Source: CAD feature listing. Evaluate the final solid. Frame: model axes, mm. A direction names the side the tool comes from. Give positions to 0.01 mm unless a question says otherwise; leave off trailing zeros. Loops run counter-clockwise (first coordinate to the right, second up) from the corner with the lowest first, then second, coordinate; pieces in that order, holes last. Notation, with made-up numbers: (48.5, -33) -> (103.5, -33) arc R28 ccw to (103.5, 2) -> close; hole circle Ø6 at (-36.5, 71). An arc over 180 degrees is marked (long way). Put each result on its own line as item: value.
Autodesk Fusion 360 part; units mm, degrees
sketch "Sketch1" plane through (0, 0, 0) normal (0, 1, 0) x (1, 0, 0)
  circle A0 centre (0, 0) radius 80
  dimension "d1" = 160
extrude "Extrude1" add sketch "Sketch1" along normal blind 10 makes body 1
fillet "Fillet1" radius 4 1 edges at (-74.5862, 10, 28.9292) on bodies 1
sketch "Sketch2" plane through (0, 0, 0) normal (0, 1, 0) x (1, 0, 0)
  line L0 (125, 0) -> (165, 0)
  line L1 (165, 0) -> (165, 120)
  line L2 (165, 120) -> (125, 120)
  line L3 (125, 120) -> (125, 0)
  circle A0 centre (145, 100) radius 2
  circle A1 centre (145, 81.9961) radius 2
  circle A2 centre (145, 50) radius 10
  point P0 (145, 100)
  dimension "d5" = 120
  dimension "d6" = 40
  dimension "d7" = 4
  dimension "d8" = 4
  dimension "d9" = 20
extrude "Extrude2" add sketch "Sketch2" along normal blind 12 separate body makes body 2
sketch "Sketch3" plane through (0, 0, 0) normal (0, 1, 0) x (1, 0, 0)
  line L0 (145, 104) -> (141.5359, 102)
  line L1 (141.5359, 102) -> (141.5359, 98)
  line L2 (141.5359, 98) -> (145, 96)
  line L3 (145, 96) -> (148.4641, 98)
  line L4 (148.4641, 98) -> (148.4641, 102)
  line L5 (148.4641, 102) -> (145, 104)
  line L6 (145, 86) -> (141.5359, 84)
  line L7 (141.5359, 84) -> (141.5359, 80)
  line L8 (141.5359, 80) -> (145, 78)
  line L9 (145, 78) -> (148.4641, 80)
  line L10 (148.4641, 80) -> (148.4641, 84)
  line L11 (148.4641, 84) -> (145, 86)
  point P0 (145, 100)
  point P1 (145, 82)
extrude "Extrude3" cut sketch "Sketch3" along normal blind 4 contours L6 L7 L8 L9 L10 L11 bodies 2
sketch "Sketch4" plane through (0, 0, 0) normal (0, 1, 0) x (1, 0, 0)
  line L0 (145, 104) -> (141.5359, 102)
  line L1 (141.5359, 102) -> (141.5359, 98)
  line L2 (141.5359, 98) -> (145, 96)
  line L3 (145, 96) -> (148.4641, 98)
  line L4 (148.4641, 98) -> (148.4641, 102)
  line L5 (148.4641, 102) -> (145, 104)
  point P0 (145, 100)
extrude "Extrude4" cut sketch "Sketch4" along normal blind 4 bodies 2
fillet "Fillet2" radius 4 1 edges at (165, 6, -120) on bodies 2
fillet "Fillet3" radius 4 1 edges at (125, 6, -120) on bodies 2
fillet "Fillet4" radius 2 1 edges at (135.6767, 12, -53.6162) on bodies 2
fillet "Fillet5" radius 2 1 edges at (135.6767, 0, -53.6162) on bodies 2
move_body "Move1" bodies 2 to x (1, 0, 0) y (0, 0, 1) z (0, -1, 0) at (0, 0, 0)
move_body "Move2" bodies 2 to x (1, 0, 0) y (0, 1, 0) z (0, 0, 1) at (0, 10, 0)
move_body "Move3" bodies 2 to x (1, 0, 0) y (0, 1, 0) z (0, 0, 1) at (-145, 0, 0)
move_body "Move4" bodies 2 to x (1, 0, 0) y (0, 1, 0) z (0, 0, 1) at (0, 0, -50)
combine "Combine1" operation add target body 1 tool bodies 2
fillet "Fillet6" radius 2 5 edges at (20, 68, -50) (18.8284, 128.8284, -50) (0, 130, -50) (-18.8284, 128.8284, -50) (-20, 68, -50) on bodies 1
fillet "Fillet7" radius 2 5 edges at (20, 68, -38) (18.8284, 128.8284, -38) (0, 130, -38) (-18.8284, 128.8284, -38) (-20, 68, -38) on bodies 1
fillet "Fillet8" radius 20 8 edges at (-19.4142, 10, -38.5858) (-20, 10, -44) (-19.4142, 10, -49.4142) (0, 10, -50) (19.4142, 10, -49.4142) (20, 10, -44) (19.4142, 10, -38.5858) (0, 10, -38) on bodies 1
(1) Section A-A on y = 60. Return loops of the section in (x, z).
Calculated:
outline: (-20, -48) arc R2 ccw to (-18, -50) -> (-12, -50) arc R2 ccw to (-10, -48) -> (-10, -40) arc R2 ccw to (-12, -38) -> (-18, -38) arc R2 ccw to (-20, -40) -> close; (10, -48) arc R2 ccw to (12, -50) -> (18, -50) arc R2 ccw to (20, -48) -> (20, -40) arc R2 ccw to (18, -38) -> (12, -38) arc R2 ccw to (10, -40) -> close
(2) First-contact query: P1, Ø5, axis at x = -62, z = 5, coming from the +Y side; P2, Ø12, axis at y = 106, z = -44, coming from the +X side; P3, Ø2, axis at x = -11.5, z = 21.5, coming from the -Y side; P4, Ø7.5, axis at x = -1.5, y = 111.5, coming from the -Z side. Flat tips, straight axial feed; report the tip coordinate or a pass-through.
Calculated:
P1: stops at y = 10
P2: stops at x = 20
P3: stops at y = 0
P4: stops at z = -50
(3) Reachability of faces 1 (the cylindrical face through (-0.252, 16.014, -32.297)), 2 (the flat face through (0, 80, -50)), 3 (the flat face through (-2, 108, -46)), 4 (the flat face through (-20, 79, -44)), 5 (the flat face through (20, 77, -44)) from +Z, -Z, +X, -X, +Y, -Y: full face, straight path, thin tool, end or side. Return the list, or none.
Calculated:
face 1: +Z, +X, -X, +Y
face 2: -Z, +X, -X, +Y
face 3: -Z
face 4: +Z, -Z, -X, +Y
face 5: +Z, -Z, +X, +Y
(4) Section D-D on y = 20.5. Return loops of the section in (x, z), then the cut area to 3 significant figures.
Calculated:
outline: (-22.4, -48) arc R4.4 ccw to (-18, -52.4) -> (18, -52.4) arc R4.4 ccw to (22.4, -48) -> (22.4, -40) arc R4.4 ccw to (18, -35.6) -> (-18, -35.6) arc R4.4 ccw to (-22.4, -40) -> close
area: 736 mm²
(5) Section B-B on y = 81. Return loops of the section in (x, z).
Calculated:
outline: (-20, -48) arc R2 ccw to (-18, -50) -> (18, -50) arc R2 ccw to (20, -48) -> (20, -40) arc R2 ccw to (18, -38) -> (-18, -38) arc R2 ccw to (-20, -40) -> close
(6) Section C-C on z = 0. Return loops of the section in (x, y), then the cut area to 3 significant figures.
Calculated:
outline: (-80, 0) -> (80, 0) -> (80, 6) arc R4 ccw to (76, 10) -> (-76, 10) arc R4 ccw to (-80, 6) -> close
area: 1,590 mm²
(7) Draft query along X for faces 6 (the flat face through (0, 80, -38)), 7 (the cylindrical face through (-18.797, 128.859, -43.944)), 8 (the cylindrical face through (-0.43, 93.95, -42.06)). Return one class per face: released by +X, released by -X, zero draft, split by the parting line, or undercut.
Calculated:
face 6: zero draft
face 7: released by -X
face 8: undercut
(8) Line query: probe 1 along Y at (x, z) = (0, -42.5); probe 2 along X at (y, z) = (110, -39.75); probe 3 along Y at (x, z) = (0, -39.5). Output: solid intervals per line, ascending. Write a range as from..to.
Calculated:
probe 1: y = 0..50, 70..90, 94..108, 112..130
probe 2: x = -19.98..-2, 2..19.98
probe 3: y = 0..49.94, 70.06..90, 94..108, 112..129.94
